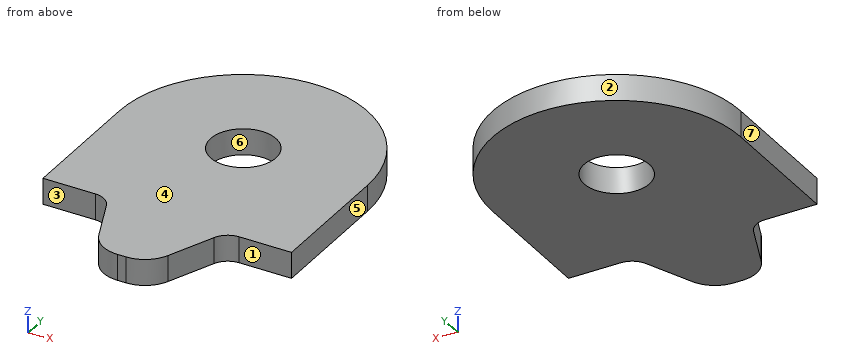
from build123d import *

# Parameters (mm, degrees)
SKETCH1_R           = 2.5
SKETCH1_R_2         = 1.5
BOSS_EXTRUDE1_DEPTH = 4
SKETCH2_R           = 5
CUT_EXTRUDE1_DEPTH  = 50.010203019
FILLET1_R           = 5
FILLET2_R           = 3


with BuildPart() as part:
    # Sketch1 → Boss-Extrude1 (new body)
    with BuildSketch(Plane.XY):
        with BuildLine():
            Line((-19, 0), (-19, -32))
            Line((-19, -32), (-14.8, -32))
            Line((-14.8, -32), (-14.8, -45))
            Line((-14.8, -45), (-5, -45))
            Line((-5, -45), (-5, -42))
            Line((-5, -42), (5, -42))
            Line((5, -42), (5, -45))
            Line((5, -45), (19, -45))
            Line((19, -45), (19, 0))
            ThreePointArc((19, 0), (0, 19), (-19, 0))
        make_face()
        Circle(SKETCH1_R, mode=Mode.SUBTRACT)
        with Locations((-14, -27)):
            Circle(SKETCH1_R_2, mode=Mode.SUBTRACT)
        with Locations(Location((14, -27, 0), (0, 0, 180))):
            Circle(SKETCH1_R_2, mode=Mode.SUBTRACT)
    extrude(amount=BOSS_EXTRUDE1_DEPTH)

    # Sketch2 → Cut-Extrude1 (cut, through all)
    with BuildSketch(Plane.XY.offset(4)):
        Circle(SKETCH2_R)
        Polygon((-19, -20), (-9, -20), (-4, -32), (4, -32), (9, -20), (19, -20), (19, -45), (-19, -45), align=None)
    extrude(amount=-CUT_EXTRUDE1_DEPTH, mode=Mode.SUBTRACT)

    # Fillet1
    fillet1_edges = [part.edges().sort_by_distance(p)[0] for p in [
        (-4, -32, 2),
        (4, -32, 2),
    ]]
    fillet(fillet1_edges, radius=FILLET1_R)

    # Fillet2
    fillet2_edges = [part.edges().sort_by_distance(p)[0] for p in [
        (-9, -20, 2),
        (9, -20, 2),
    ]]
    fillet(fillet2_edges, radius=FILLET2_R)


solid = part.part
Input: part model. Units: mm. Frame: model coordinates. Face numbers are marked on the shaded views. A direction names the side the tool comes from. Coordinates: 2 decimals unless noted, no trailing zeros. Order: outer loops, then holes, each group sorted by start corner. A loop starts at its lowest first (then second) coordinate and runs counter-clockwise, first axis right, second up.
1. Cut plane D-D, the plane y = -23. Return loops of the section in (x, z).
Checked values:
outline: (-7.75, 0) - (7.75, 0) - (7.75, 4) - (-7.75, 4) - close
2. Contact query for a flat-ended pin moving along its axis: P1, Ø2, axis at y = -26, z = 1.5, coming from the -X side. Output: stop coordinate, or through.
Checked values:
P1: stops at x = -6.92
3. Cut plane C-C, the plane y = 4. Return loops of the section in (x, z), plus the area to 3 significant figures.
Checked values:
outline: (-18.57, 0) - (-3, 0) - (-3, 4) - (-18.57, 4) - close; (3, 0) - (18.57, 0) - (18.57, 4) - (3, 4) - close
area: 125 mm2
4. Cut plane A-A, the plane x = 0. Return loops of the section in (y, z).
Checked values:
outline: (-32, 0) - (-5, 0) - (-5, 4) - (-32, 4) - close; (5, 0) - (19, 0) - (19, 4) - (5, 4) - close
5. Draft query along X for the marked faces 4, 5, 6 and 7. Return one class per face: +X half, -X half, draft (parallel to the pull), parting line (faces both ways), or undercut.
Checked values:
face 4: draft
face 5: +X half
face 6: undercut
face 7: -X half
6. Ray query, line 1 along Y through (x, z) = (0, 2.85); line 2 along Y through (x, z) = (-2, 1.1); line 3 along X through (y, z) = (-3.5, 2.65). Return the intervals inside material, ascending.
Checked values:
line 1: y = -32 to -5, 5 to 19
line 2: y = -31.82 to -4.58, 4.58 to 18.89
line 3: x = -19 to -3.57, 3.57 to 19
7. Access query for the marked faces 1, 2 and 3. Directions: +Z, -Z, +X, -X, +Y, -Y. A direction counts if a zero-diameter tool reaches every point of the face in a straight line with its end or side. Return the directions, or none.
Checked values:
face 1: +Z, -Z, +X, -Y
face 2: +Z, -Z, +Y
face 3: +Z, -Z, -X, -Y
8. Cut plane B-B, the plane z = 2.9. Return loops of the section in (x, y), plus the area to 3 significant figures.
Checked values:
outline: (-19, -20) - (-11, -20) arc R3 cw to (-8.23, -21.85) - (-5.28, -28.92) arc R5 ccw to (-0.67, -32) - (0.67, -32) arc R5 ccw to (5.28, -28.92) - (8.23, -21.85) arc R3 cw to (11, -20) - (19, -20) - (19, 0) arc R19 ccw to (-19, 0) - close; hole circle Ø10 at (0, 0)
area: 1,400 mm2
